```python
from build123d import *

# Parameters (mm, degrees)
F1_R     = 4
F3_DEPTH = 12.5


with BuildPart() as f2:
    # F0 (on Front) → F2 (revolve)
    with BuildSketch(Plane.XZ):
        Polygon((0, 11), (0, 0), (7, 0), (7, 15), (5, 15), (1.5, 11), align=None)
        Polygon((-7, 0), (0, 0), (0, 11), (-1.5, 11), (-5, 15), (-7, 15), align=None)
    revolve(axis=Axis((0, 0, 0), (1, 0, 0)))

    # F1 (on Right) → F3 (cut, symmetric)
    with BuildSketch(Plane.YZ):
        Circle(F1_R)
    extrude(amount=F3_DEPTH, both=True, mode=Mode.SUBTRACT)


solid = f2.part
```
Model file for the job. Use its own axes, mm. A direction names the side the tool comes from. Round coordinates to 2 decimals unless told otherwise and drop trailing zeros. Loops run counter-clockwise (first coordinate to the right, second up) from the corner with the lowest first, then second, coordinate; pieces in that order, holes last. Notation, with made-up numbers: M 17,66.25 L 33,66.25 A11 cw 33,79.25 Z; hole C 47.5,70 d10. An arc over 180 degrees is marked long. Put each result on its own line as item: value. Start each with the question number.
Item 1: Cut at C-C (x = -4.5). List the corners of the cut face in (y, z).
Item 2: Cut at A-A (z = 0). List the corners of the cut face in (x, y).
Item 3: Cut at D-D (x = 2.75). List the corners of the cut face in (y, z).
Item 4: Drop flat-ended pins along their axis: P1, Ø8, axis at x = 1.5, z = 7.5, coming from the -Y side; P2, Ø6, axis at x = -3.5, y = -7.5, coming from the +Z side; P3, Ø5, axis at x = 3.5, z = -3, coming from the -Y side. Give the stop position or say it passes through.
Item 5: 3-axis set-ups, long thin cutter, end or side, ignore diameter. For faces 4 (the face through (-6.014, -0.66, -14.985)), 5 (the face through (1.67, 10.93, -2.43)): which of +Z, -Z, +X, -X, +Y, -Y reach the whole face in a straight line?
Item 6: Mould opens along Y. For faces 1 (the face through (0.098, -0.867, -3.905)), 2 (the face through (-7, 3, 3)), 3 (the face through (-1.7, -3.4, 10.7)) say: released by +Y, released by -Y, zero draft, split by the parting line, or undercut.
Item 7: Drill centre lines: line 1 along Z through (x, y) = (-1.5, 0); line 2 along X through (y, z) = (13, -1.25); line 3 along Z through (x, y) = (-5.75, 0.25). Where is each one in solid material? Low to high.
Answer block:
1. outline: C 0,0 d28.86; hole C 0,0 d8
2. outline: M -7,-15 L -5,-15 L -1.5,-11 L 1.5,-11 L 5,-15 L 7,-15 L 7,-4 L -7,-4 Z; M -7,4 L 7,4 L 7,15 L 5,15 L 1.5,11 L -1.5,11 L -5,15 L -7,15 Z
3. outline: C 0,0 d24.86; hole C 0,0 d8
4. P1: y = -13.93
4. P2: z = 14.18
4. P3: y = -14.97
5. face 4: +X, -X
5. face 5: none
6. face 1: undercut
6. face 2: zero draft
6. face 3: split by the parting line
7. line 1: -11 to -4, 4 to 11
7. line 2: -7 to -3.3, 3.3 to 7
7. line 3: -15 to -3.99, 3.99 to 15
